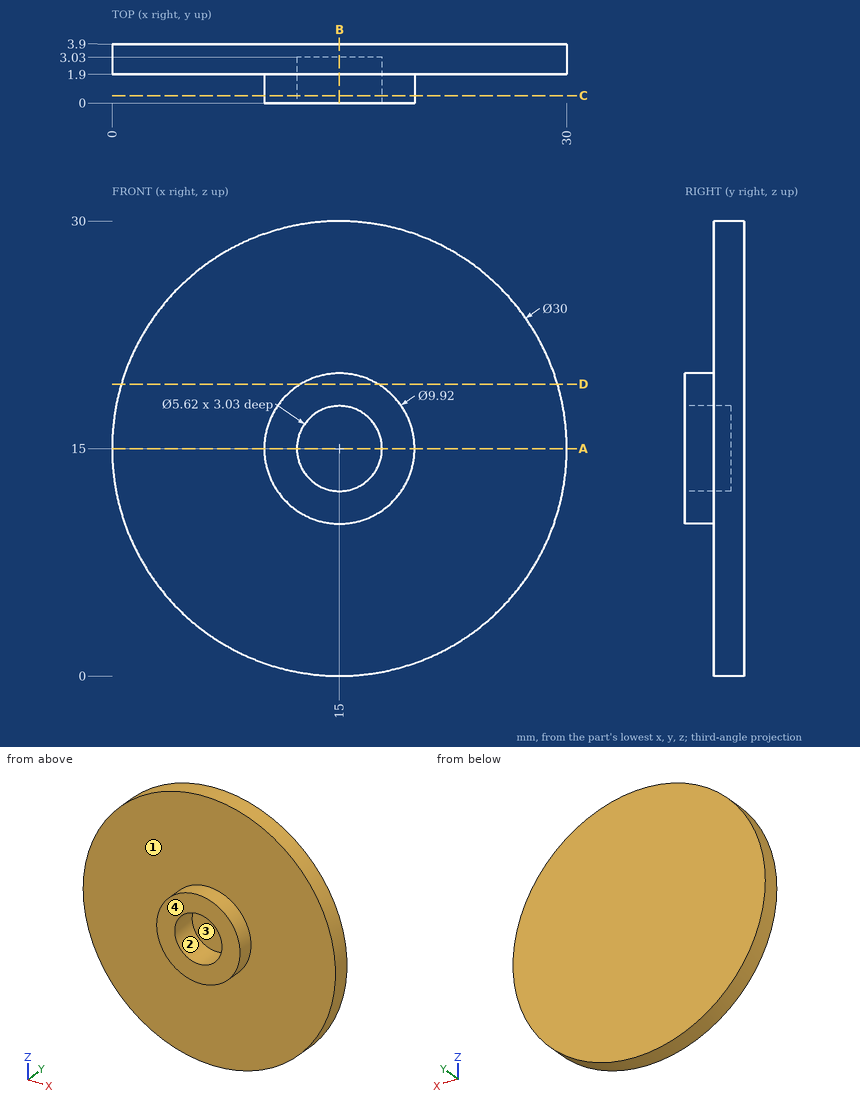
Design review of the part shown in the three views and the two pictorial views. Dimensions are in mm from the part's minimum x, y and z. A direction names the side the tool comes from. Coordinates: 2 decimals unless noted, no trailing zeros. Write each loop counter-clockwise with the first axis right and the second up, starting at its lowest first coordinate (ties: lowest second). Pieces come first, ordered by that corner, then holes. Notation, with made-up numbers: (-17, 26.5) -> (0, 26.5) arc R22 cw to (0, 62.5) -> close; hole circle Ø10 at (-36.75, 44). An arc over 180 degrees is marked (long way). Answer in a Markdown table with one row per item.
1. We need section A-A, the plane z = 15. State the section outline as (x, y) points.
Answers below:
| item | result |
|---|---|
| outline | (0, 1.9) -> (10.04, 1.9) -> (10.04, 0) -> (12.19, 0) -> (12.19, 3.03) -> (17.81, 3.03) -> (17.81, 0) -> (19.96, 0) -> (19.96, 1.9) -> (30, 1.9) -> (30, 3.9) -> (0, 3.9) -> close |
2. Draft analysis for pull direction Z (two halves, no side actions). For the marked faces 1 and 2, state which applies: +Z half, -Z half, draft (parallel to the pull), parting line (faces both ways), or undercut.
Answers below:
| item | result |
|---|---|
| face 1 | draft |
| face 2 | undercut |
3. We need section B-B, the plane x = 15. State the section outline as (y, z) points, and give its area (3 significant figures).
Answers below:
| item | result |
|---|---|
| outline | (0, 10.04) -> (1.9, 10.04) -> (1.9, 0) -> (3.9, 0) -> (3.9, 30) -> (1.9, 30) -> (1.9, 19.96) -> (0, 19.96) -> (0, 17.81) -> (3.03, 17.81) -> (3.03, 12.19) -> (0, 12.19) -> close |
| area | 61.8 mm^2 |
4. Clearance check with flat-ended pins moving along their axes: pin 1 Ø1 at (x, y) = (22, 1) entering from +Z; pin 2 Ø8 at (x, z) = (17.5, 25) entering from -Y. State where each tip first meets the part, or that it passes through.
Answers below:
| item | result |
|---|---|
| pin 1 | passes through |
| pin 2 | stops at y = 1.9 |
5. We need section D-D, the plane z = 19.25. State the section outline as (x, y) points.
Answers below:
| item | result |
|---|---|
| outline | (0.61, 1.9) -> (12.44, 1.9) -> (12.44, 0) -> (17.56, 0) -> (17.56, 1.9) -> (29.39, 1.9) -> (29.39, 3.9) -> (0.61, 3.9) -> close |
6. We need section C-C, the plane y = 0.5. State the section outline as (x, z) points, and give its area (3 significant figures).
Answers below:
| item | result |
|---|---|
| outline | circle Ø9.92 at (15, 15); hole circle Ø5.62 at (15, 15) |
| area | 52.5 mm^2 |
7. For the marked faces 3 and 4, list the 3-axis set-ups (+Z, -Z, +X, -X, +Y, -Y) from which the entire face can be reached by the end or side of a thin tool; tool diameter is ignored.
Answers below:
| item | result |
|---|---|
| face 3 | -Y |
| face 4 | +Z, -Z, +X, -X, -Y |
8. Wall thickness on probe 1 along Z at (x, y) = (15, 0.9); probe 2 along Z at (x, y) = (15, 2); probe 3 along Y at (x, z) = (25.5, 23): over which ranges is each line inside the solid? List them lowest first. Write a range as [from, to].
Answers below:
| item | result |
|---|---|
| probe 1 | z = [10.04, 12.19], [17.81, 19.96] |
| probe 2 | z = [0, 12.19], [17.81, 30] |
| probe 3 | y = [1.9, 3.9] |
